```python
from build123d import *

# Parameters (mm, degrees)
SKETCH1_W             = 76.2
SKETCH1_H             = 19.05
BOSS_EXTRUDE1_DEPTH   = 1.6
BOSS_EXTRUDE2_DEPTH   = 1.6
BOSS_EXTRUDE3_DEPTH   = 1.6
BOSS_EXTRUDE4_DEPTH   = 1.6
BOSS_EXTRUDE5_DEPTH   = 1.6
FILLET4_R             = 1.5875
F_4_CLEARANCE_HOLE1_D = 2.9464


with BuildPart() as part:
    # Sketch1 → Boss-Extrude1 (new body)
    with BuildSketch(Plane(origin=(0, 0, 0), x_dir=(1, 0, 0), z_dir=(0, 1, 0))):
        Rectangle(SKETCH1_W, SKETCH1_H)
    extrude(amount=BOSS_EXTRUDE1_DEPTH)

    # Sketch2 → Boss-Extrude2 (add)
    with BuildSketch(Plane.XZ):
        Polygon((-40.48125, -13.649445986), (-29.089234633, -20.226629124), (-22.910646178, -9.525), (-34.302661544, -2.947816861), align=None)
    boss_extrude2 = extrude(amount=-BOSS_EXTRUDE2_DEPTH)

    # Sketch3 → Boss-Extrude3 (add)
    with BuildSketch(Plane.XZ):
        Polygon((-38.1, 9.525), (-40.48125, -13.649445986), (-22.910646178, -9.525), align=None)
    boss_extrude3 = extrude(amount=-BOSS_EXTRUDE3_DEPTH)

    # Mirror1: Boss-Extrude2, Boss-Extrude3 across plane
    add(boss_extrude2.mirror(Plane(origin=(0, 0, 0), x_dir=(0, 0, 1), z_dir=(1, 0, 0))))
    add(boss_extrude3.mirror(Plane(origin=(0, 0, 0), x_dir=(0, 0, 1), z_dir=(1, 0, 0))))

    # Sketch4 → Boss-Extrude4 (add)
    with BuildSketch(Plane.XZ):
        with BuildLine():
            Line((-29.089234633, -20.226629124), (-29.089234633, 9.525))
            Line((-29.089234633, 9.525), (29.089234633, 9.525))
            Line((29.089234633, 9.525), (29.089234633, -20.226629124))
            ThreePointArc((29.089234633, -20.226629124), (0, -9.525), (-29.089234633, -20.226629124))
        make_face()
    extrude(amount=-BOSS_EXTRUDE4_DEPTH)

    # Sketch5 → Boss-Extrude5 (add)
    with BuildSketch(Plane.XZ):
        Polygon((-38.1, 9.525), (-37.969503353, 10.795), (37.969503353, 10.795), (38.1, 9.525), align=None)
    extrude(amount=-BOSS_EXTRUDE5_DEPTH)

    # Fillet4
    fillet4_edges = [part.edges().sort_by_distance(p)[0] for p in [
        (-40.48125, 0.8, -13.649445986),
        (-29.089234633, 0.8, -20.226629124),
        (40.48125, 0.8, -13.649445986),
        (29.089234633, 0.8, -20.226629124),
        (37.969503353, 0.8, 10.795),
        (-37.969503353, 0.8, 10.795),
    ]]
    fillet(fillet4_edges, radius=FILLET4_R)

    # #4 Clearance Hole1 (through all)
    with Locations(Plane(origin=(-22.225, 0, 4.621670802), x_dir=(0, 0, -1), z_dir=(0, -1, 0))):
        with Locations((0, 0), (8.248891971, -4.7625), (16.497783942, -9.525)):
            f_4_clearance_hole1 = Hole(F_4_CLEARANCE_HOLE1_D / 2)

    # Mirror2: #4 Clearance Hole1 across plane
    add(f_4_clearance_hole1.mirror(Plane(origin=(0, 0, 0), x_dir=(0, 0, 1), z_dir=(1, 0, 0))), mode=Mode.SUBTRACT)


solid = part.part
```
The listing builds one solid part. Answer for the finished solid, in the listing's coordinates (mm). Give positions to 0.01 mm unless a question says otherwise; leave off trailing zeros. Order: outer loops, then holes, each group sorted by start corner. A loop starts at its lowest first (then second) coordinate and runs counter-clockwise, first axis right, second up.
1) Determine the mould class of faces 1 (the face through (-25.527, 0.811, -3.819)), 2 (the face through (0.428, 0.789, -9.527)), 3 (the face through (-1, 1, 10.795)) for opening direction Z: pulls with the +Z half, pulls with the -Z half, needs draft (parallel to the pull), parting line crosses it, or undercut.
Reported:
face 1: undercut
face 2: pulls with the -Z half
face 3: pulls with the +Z half
2) Find section D-D on y = 0.7. Give the number of separate pieces and of enclosed holes in the cut face, then the cut area to 3 significant figures.
Reported:
separate pieces: 1
enclosed holes: 6
area: 1,910 mm2
3) Consider line 1 along X through (y, z) = (1.3, -3.5); line 2 along X through (y, z) = (1.5, 3.5); line 3 along Z through (x, y) = (-28, 0.55) (3 decimals). Determine where each line is inside the solid, lowest interval first.
Reported:
line 1: x = -39.44 to -28.46, -25.52 to 25.52, 28.46 to 39.44
line 2: x = -38.72 to -23.18, -21.27 to 21.27, 23.18 to 38.72
line 3: z = -19.329 to -4.697, -2.557 to 10.795
4) Find section A-A on z = -18. Write down the section's boundary in (x, y), then the cut area to 3 significant figures.
Reported:
outline: (-32.95, 0) - (-26.25, 0) - (-26.25, 1.6) - (-32.95, 1.6) - close; (26.25, 0) - (32.95, 0) - (32.95, 1.6) - (26.25, 1.6) - close
area: 21.4 mm2
5) Find section B-B on x = -31.75. Write down the section's boundary in (y, z) (3 decimals).
Reported:
outline: (0, -18.69) - (1.6, -18.69) - (1.6, -13.349) - (0, -13.349) - close; (0, -10.403) - (1.6, -10.403) - (1.6, 10.795) - (0, 10.795) - close
6) Find section C-C on z = 5. Write down the section's boundary in (x, y), then the cut area to 3 significant figures.
Reported:
outline: (-38.56, 0) - (-23.65, 0) - (-23.65, 1.6) - (-38.56, 1.6) - close; (-20.8, 0) - (20.8, 0) - (20.8, 1.6) - (-20.8, 1.6) - close; (23.65, 0) - (38.56, 0) - (38.56, 1.6) - (23.65, 1.6) - close
area: 114 mm2
